```python
from build123d import *

# Parameters (mm, degrees)
BOSS_EXTRUDE1_DEPTH     = 50.8
SKETCH2_R               = 2.667
CUT_EXTRUDE1_DEPTH      = 23.225
CUT_EXTRUDE1_DEPTH_BACK = 4.175
SKETCH3_R               = 2.667
CUT_EXTRUDE2_DEPTH      = 3.175
FILLET1_R               = 1.27
FILLET2_R               = 1.27


with BuildPart() as part:
    # Sketch1 → Boss-Extrude1 (new body)
    with BuildSketch(Plane.XY):
        Polygon((0, -22.225), (22.225, -22.225), (22.225, -25.4), (-3.175, -25.4), (-3.175, 0), (0, 0), align=None)
    extrude(amount=BOSS_EXTRUDE1_DEPTH)

    # Sketch2 → Cut-Extrude1 (cut, two sides)
    with BuildSketch(Plane(origin=(0, 0, 0), x_dir=(0, 0, -1), z_dir=(1, 0, 0))) as cut_extrude1_sk:
        with Locations((-38.1, -17.653)):
            Circle(SKETCH2_R)
        with Locations((-12.7, -17.653)):
            Circle(SKETCH2_R)
    extrude(amount=CUT_EXTRUDE1_DEPTH, mode=Mode.SUBTRACT)
    extrude(cut_extrude1_sk.sketch, amount=-CUT_EXTRUDE1_DEPTH_BACK, mode=Mode.SUBTRACT)

    # Sketch3 → Cut-Extrude2 (cut)
    with BuildSketch(Plane(origin=(0, -22.225, 0), x_dir=(1, 0, 0), z_dir=(0, 1, 0))):
        with Locations((8.763, -44.45)):
            Circle(SKETCH3_R)
        with Locations((8.763, -31.75)):
            Circle(SKETCH3_R)
        with Locations((8.763, -19.05)):
            Circle(SKETCH3_R)
        with Locations((8.763, -6.35)):
            Circle(SKETCH3_R)
    extrude(amount=-CUT_EXTRUDE2_DEPTH, mode=Mode.SUBTRACT)

    # Fillet1
    fillet1_edges = [part.edges().sort_by_distance(p)[0] for p in [
        (0, -22.225, 25.4),
    ]]
    fillet(fillet1_edges, radius=FILLET1_R)

    # Fillet2
    fillet2_edges = [part.edges().sort_by_distance(p)[0] for p in [
        (-3.175, -25.4, 25.4),
    ]]
    fillet(fillet2_edges, radius=FILLET2_R)


solid = part.part
```
The listing builds one solid part. Answer for the finished solid, in the listing's coordinates (mm). A direction names the side the tool comes from. Coordinates: 2 decimals unless noted, no trailing zeros. Loops run counter-clockwise (first coordinate to the right, second up) from the corner with the lowest first, then second, coordinate; pieces in that order, holes last. Notation, with made-up numbers: (13.25, 0.5) - (60.25, 0.5) arc R19 cw to (60.25, 36.5) - close; hole circle Ø5 at (-8.5, 65). An arc over 180 degrees is marked (long way). Use a Markdown table: item, result. Add a question column.
1) The part is cut by section D-D, the plane x = -1.25. Give the vertices of the cut face in (y, z).
2) Given pin 1 (7 mm diameter, centred on x = 8.763, z = 19.05, fed in from +Y) (3 decimals); pin 2 (4.5 mm diameter, centred on x = 8.763, z = 31.75, fed in from -Y); pin 3 (6 mm diameter, centred on y = -17.653, z = 12.7, fed in from +X), each flat-ended and moving along its own axis, determine where each tip first touches the part or whether it passes through.
3) For faces 4 (the flat face through (0, -10, 25)), 5 (the cylindrical face through (8.416, -23.79, 41.806)), determine the directions among +Z, -Z, +X, -X, +Y, -Y from which every point of the face is accessible in a straight line to the end or side of a thin tool.
4) Find the intervals of material crossed by line 1 (X direction, y = -24.15, z = 19.05) (3 decimals); line 2 (Y direction, x = -1.4, z = 38.1); line 3 (X direction, y = -20, z = 28) (3 decimals), in increasing order.
5) The part is cut by section A-A, the plane z = 31.75. Give the vertices of the cut face in (x, y) (3 decimals), and give its area (3 significant figures).
6) The part is cut by section C-C, the plane z = 25. Give the vertices of the cut face in (x, y) (3 decimals), and give its area (3 significant figures).
7) The part is cut by section B-B, the plane x = 10. Give the vertices of the cut face in (y, z) (3 decimals), and give its area (3 significant figures).
8) The mould has two halves that part along Z. Classify faces 1 (the flat face through (5, -23, 50.8)), 2 (the cylindrical face through (11.307, -23.79, 5.549)), 3 (the flat face through (-3.175, -12, 25)): released by +Z, released by -Z, zero draft, split by the parting line, or undercut.
Here are the results:
| question | item | result |
|---|---|---|
| 1 | outline | (-25.4, 0) - (0, 0) - (0, 50.8) - (-25.4, 50.8) - close; hole circle Ø5.33 at (-17.65, 12.7); hole circle Ø5.33 at (-17.65, 38.1) |
| 2 | pin 1 | stops at y = -22.225 |
| 2 | pin 2 | passes through |
| 2 | pin 3 | stops at x = 0 |
| 3 | face 4 | +Z, -Z, +X, +Y |
| 3 | face 5 | +Y, -Y |
| 4 | line 1 | x = -3.175 to 6.096, 11.43 to 22.225 |
| 4 | line 2 | y = -25.4 to -20.32, -14.99 to 0 |
| 4 | line 3 | x = -3.175 to 0 |
| 5 | outline | (-3.175, -24.13) arc R1.27 ccw to (-1.905, -25.4) - (6.096, -25.4) - (6.096, -22.225) - (1.27, -22.225) arc R1.27 cw to (0, -20.955) - (0, 0) - (-3.175, 0) - close; (11.43, -25.4) - (22.225, -25.4) - (22.225, -22.225) - (11.43, -22.225) - close |
| 5 | area | 134 mm^2 |
| 6 | outline | (-3.175, -24.13) arc R1.27 ccw to (-1.905, -25.4) - (22.225, -25.4) - (22.225, -22.225) - (1.27, -22.225) arc R1.27 cw to (0, -20.955) - (0, 0) - (-3.175, 0) - close |
| 6 | area | 151 mm^2 |
| 7 | outline | (-25.4, 0) - (-22.225, 0) - (-22.225, 3.987) - (-25.4, 3.987) - close; (-25.4, 8.713) - (-22.225, 8.713) - (-22.225, 16.687) - (-25.4, 16.687) - close; (-25.4, 21.413) - (-22.225, 21.413) - (-22.225, 29.387) - (-25.4, 29.387) - close; (-25.4, 34.113) - (-22.225, 34.113) - (-22.225, 42.087) - (-25.4, 42.087) - close; (-25.4, 46.813) - (-22.225, 46.813) - (-22.225, 50.8) - (-25.4, 50.8) - close |
| 7 | area | 101 mm^2 |
| 8 | face 1 | released by +Z |
| 8 | face 2 | undercut |
| 8 | face 3 | zero draft |
